Geometry: final body of the model. Coordinates: model frame, mm. A direction names the side the tool comes from. Give positions to 0.01 mm unless a question says otherwise; leave off trailing zeros. Write each loop counter-clockwise with the first axis right and the second up, starting at its lowest first coordinate (ties: lowest second). Pieces come first, ordered by that corner, then holes. Notation, with made-up numbers: (25.25, 83) -> (45.25, 83) arc R23 cw to (45.25, 107) -> close; hole circle Ø3 at (-9, 58.25). An arc over 180 degrees is marked (long way). Answer as a JSON object with one key per item and string values. Group by question number.
(1) Section query A-A on x = 35. Output: boundary loops of the cut face in (y, z), plus the area to 3 significant figures.
(2) Material intervals for probe 1 along Z at (x, y) = (7.5, 9); probe 2 along Y at (x, z) = (29, -10); probe 3 along Y at (x, z) = (24, -6.5), sorted ascending.
(3) Set-up query: faces 4 (the face through (25, 4.572, 3)), 5 (the face through (25, 4.572, -7)), 6 (the face through (49, 9.652, -2)). Return all of +Z, -Z, +X, -X, +Y, -Y with unobstructed straight access to the full face (end or side cutting, diameter ignored); none if empty.
(4) Section query B-B on y = 15.75. Output: boundary loops of the cut face in (x, z).
(5) Section query C-C on z = 6.25. Output: boundary loops of the cut face in (x, y), plus the area to 3 significant figures.
(6) Contact query for flat-ended pins moving along their axis: pin 1 Ø1.1 at (x, z) = (48, 0) entering from +Y; pin 2 Ø0.8 at (x, z) = (41.5, 5.5) entering from +Y; pin 3 Ø4 at (y, z) = (10, -9) entering from -X. Output: stop coordinate, or through.
(7) Draft query along X for faces 1 (the face through (42, 12.192, 6)), 2 (the face through (0, 5, -1)), 3 (the face through (2, 9.652, -2)). Return one class per face: +X half, -X half, draft (parallel to the pull), parting line (faces both ways), or undercut.
(8) Section query D-D on y = 8.5. Output: boundary loops of the cut face in (x, z).
from build123d import *

# Parameters (mm, degrees)
BOSS_EXTRUDE1_DEPTH = 50.8
SKETCH2_W           = 50.8
SKETCH2_H           = 6.096
BOSS_EXTRUDE2_DEPTH = 5.08
SKETCH3_W           = 43.18
SKETCH3_H           = 7.112
SKETCH3_H_2         = 6.096
BOSS_EXTRUDE3_DEPTH = 10.16
SKETCH4_R           = 1.4097
CUT_EXTRUDE1_DEPTH  = 7.62


with BuildPart() as part:
    # Sketch1 → Boss-Extrude1 (new body)
    with BuildSketch(Plane(origin=(0, 0, 0), x_dir=(0, 0, -1), z_dir=(1, 0, 0))):
        Polygon((0, 0), (3.048, 0), (8.509, 4.572), (-5.461, 4.572), align=None)
    extrude(amount=BOSS_EXTRUDE1_DEPTH)

    # Sketch2 → Boss-Extrude2 (add)
    with BuildSketch(Plane(origin=(0, 4.572, 0), x_dir=(1, 0, 0), z_dir=(0, 1, 0))):
        with Locations((25.4, 1.524)):
            Rectangle(SKETCH2_W, SKETCH2_H)
    extrude(amount=BOSS_EXTRUDE2_DEPTH)

    # Sketch3 → Boss-Extrude3 (add)
    with BuildSketch(Plane(origin=(0, 9.652, 0), x_dir=(1, 0, 0), z_dir=(0, 1, 0))):
        with Locations((25.4, 8.128)):
            Rectangle(SKETCH3_W, SKETCH3_H)
        with Locations((25.4, -5.08)):
            Rectangle(SKETCH3_W, SKETCH3_H)
        with Locations((25.4, 1.524)):
            Rectangle(SKETCH3_W, SKETCH3_H_2)
    extrude(amount=BOSS_EXTRUDE3_DEPTH)

    # Sketch4 → Cut-Extrude1 (cut)
    with BuildSketch(Plane(origin=(0, 19.812, 0), x_dir=(1, 0, 0), z_dir=(0, 1, 0))):
        with Locations(Location((41.91, -5.588, 0), (0, 0, 270))):
            Circle(SKETCH4_R)
        with Locations(Location((8.89, 8.636, 0), (0, 0, 270))):
            Circle(SKETCH4_R)
    extrude(amount=-CUT_EXTRUDE1_DEPTH, mode=Mode.SUBTRACT)


solid = part.part
Answer list:
{
 "1": {"outline": "(0, -3.05) -> (4.57, -8.51) -> (4.57, -4.57) -> (9.65, -4.57) -> (9.65, -11.68) -> (19.81, -11.68) -> (19.81, 8.64) -> (9.65, 8.64) -> (9.65, 1.52) -> (4.57, 1.52) -> (4.57, 5.46) -> (0, 0) -> close", "area": "276 mm2"},
 "2": {"probe 1": "-4.57 to 1.52", "probe 2": "9.65 to 19.81", "probe 3": "2.89 to 4.57, 9.65 to 19.81"},
 "3": {"face 4": "+Z, +X, -X", "face 5": "-Z, +X, -X", "face 6": "+Z, -Z, +X, +Y"},
 "4": {"outline": "(3.81, -11.68) -> (46.99, -11.68) -> (46.99, 8.64) -> (3.81, 8.64) -> close; hole circle Ø2.82 at (8.89, -8.64); hole circle Ø2.82 at (41.91, 5.59)"},
 "5": {"outline": "(3.81, 9.65) -> (46.99, 9.65) -> (46.99, 19.81) -> (43.15, 19.81) -> (43.15, 12.19) -> (40.67, 12.19) -> (40.67, 19.81) -> (3.81, 19.81) -> close", "area": "420 mm2"},
 "6": {"pin 1": "y = 9.65", "pin 2": "y = 12.19", "pin 3": "x = 3.81"},
 "7": {"face 1": "undercut", "face 2": "-X half", "face 3": "draft"},
 "8": {"outline": "(0, -4.57) -> (50.8, -4.57) -> (50.8, 1.52) -> (0, 1.52) -> close"}
}
